from build123d import *

# Parameters (mm, degrees)
IZIM1_W               = 1440
IZIM1_H               = 440
TABAN_FLAN_1_DEPTH    = 10
IZIM2_W               = 455
IZIM2_H               = 300
KES_EKSTR_ZYON1_DEPTH = 10
IZIM4_R               = 4.5
KES_EKSTR_ZYON4_DEPTH = 10
IZIM5_R               = 5.75
KES_EKSTR_ZYON5_DEPTH = 10


# Sheet-metal steps are written as plain solids
with BuildPart() as part:
    # Çizim1 → Taban-Flanş1 (new body)
    with BuildSketch(Plane(origin=(0, 0, 0), x_dir=(1, 0, 0), z_dir=(0, 1, 0))):
        Rectangle(IZIM1_W, IZIM1_H)
    extrude(amount=-TABAN_FLAN_1_DEPTH)

    # Çizim2 → Kes-Ekstrüzyon1 (cut)
    with BuildSketch(Plane(origin=(0, -10, 0), x_dir=(-1, 0, 0), z_dir=(0, -1, 0))):
        with Locations((310.25, 0)):
            Rectangle(IZIM2_W, IZIM2_H)
    extrude(amount=-KES_EKSTR_ZYON1_DEPTH, mode=Mode.SUBTRACT)

    # Çizim4 → Kes-Ekstrüzyon4 (cut)
    with BuildSketch(Plane(origin=(0, -10, 0), x_dir=(-1, 0, 0), z_dir=(0, -1, 0))):
        with Locations(Location((555.25, -115, 0), (0, 0, 90))):
            Circle(IZIM4_R)
        with Locations(Location((522.75, -167.5, 0), (0, 0, 90))):
            Circle(IZIM4_R)
        with Locations(Location((310.25, -167.5, 0), (0, 0, 90))):
            Circle(IZIM4_R)
        with Locations(Location((97.75, -167.5, 0), (0, 0, 90))):
            Circle(IZIM4_R)
        with Locations(Location((65.25, -115, 0), (0, 0, 90))):
            Circle(IZIM4_R)
        with Locations(Location((65.25, 115, 0), (0, 0, 270))):
            Circle(IZIM4_R)
        with Locations(Location((97.75, 167.5, 0), (0, 0, 270))):
            Circle(IZIM4_R)
        with Locations(Location((310.25, 167.5, 0), (0, 0, 270))):
            Circle(IZIM4_R)
        with Locations(Location((522.75, 167.5, 0), (0, 0, 270))):
            Circle(IZIM4_R)
        with Locations(Location((555.25, 115, 0), (0, 0, 270))):
            Circle(IZIM4_R)
    extrude(amount=-KES_EKSTR_ZYON4_DEPTH, mode=Mode.SUBTRACT)

    # Çizim5 → Kes-Ekstrüzyon5 (cut)
    with BuildSketch(Plane(origin=(0, 0, 0), x_dir=(1, 0, 0), z_dir=(0, 1, 0))):
        with Locations(Location((252.25, -12.5, 0), (0, 0, 270))):
            Circle(IZIM5_R)
        with Locations(Location((252.25, 122.5, 0), (0, 0, 270))):
            Circle(IZIM5_R)
        with Locations(Location((417.25, 122.5, 0), (0, 0, 270))):
            Circle(IZIM5_R)
        with Locations(Location((417.25, -12.5, 0), (0, 0, 270))):
            Circle(IZIM5_R)
    extrude(amount=-KES_EKSTR_ZYON5_DEPTH, mode=Mode.SUBTRACT)


solid = part.part
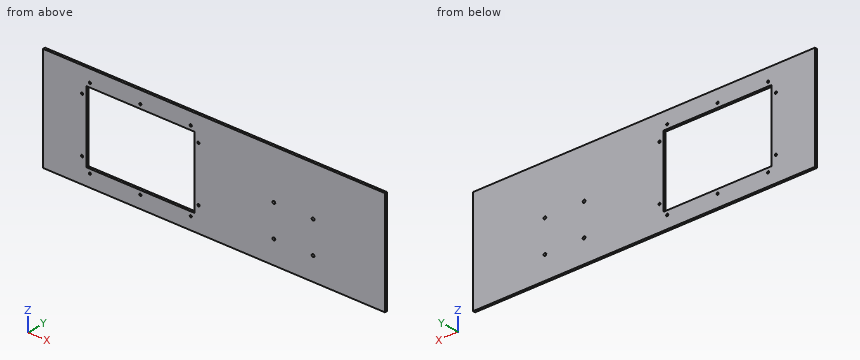
Model file for the job. Use its own axes, mm. Give positions to 0.01 mm unless a question says otherwise; leave off trailing zeros. Loops run counter-clockwise (first coordinate to the right, second up) from the corner with the lowest first, then second, coordinate; pieces in that order, holes last.
Item 1: Drill centre lines: line 1 along X through (y, z) = (-4.5, -167.5); line 2 along X through (y, z) = (-4.5, 12.5); line 3 along X through (y, z) = (-6.5, 81). Where is each one in solid material? Low to high.
Check values:
line 1: x = -720 to -527.25, -518.25 to -314.75, -305.75 to -102.25, -93.25 to 720
line 2: x = -720 to -537.75, -82.75 to 246.5, 258 to 411.5, 423 to 720
line 3: x = -720 to -537.75, -82.75 to 720
Item 2: Slice it at C-C (y = -7.25). Give the number of separate pieces and of enclosed holes in the cut face, plus the area to 3 significant figures.
Check values:
separate pieces: 1
enclosed holes: 15
area: 496,000 mm2
Item 3: Slice it at A-A (x = -249). Write the cut outline in (y, z).
Check values:
outline: (-10, -220) - (0, -220) - (0, -150) - (-10, -150) - close; (-10, 150) - (0, 150) - (0, 220) - (-10, 220) - close
Item 4: Slice it at B-B (z = 51.5). Write the cut outline in (x, y).
Check values:
outline: (-720, -10) - (-537.75, -10) - (-537.75, 0) - (-720, 0) - close; (-82.75, -10) - (720, -10) - (720, 0) - (-82.75, 0) - close
